```python
from build123d import *

# Parameters (mm, degrees)
SKETCH2_R           = 5
BOSS_EXTRUDE1_DEPTH = 10
FILLET1_R           = 3
BOSS_EXTRUDE2_DEPTH = 10
SKETCH5_R           = 5
SKETCH5_R_2         = 4.5
BOSS_EXTRUDE3_DEPTH = 10
SKETCH6_R           = 2
CUT_EXTRUDE1_DEPTH  = 10
SKETCH7_R           = 3
CUT_EXTRUDE2_DEPTH  = 10
SKETCH8_R           = 4.65
CUT_EXTRUDE3_DEPTH  = 17
SKETCH9_R           = 4.65
SKETCH9_R_2         = 5.25
CUT_EXTRUDE4_DEPTH  = 10
SKETCH9_3_R         = 1.45
CUT_EXTRUDE5_DEPTH  = 10


with BuildPart() as part:
    # Sketch2 → Boss-Extrude1 (new body)
    with BuildSketch(Plane(origin=(0, 0, 0), x_dir=(1, 0, 0), z_dir=(0, 1, 0))):
        with BuildLine():
            Line((36.25, 10), (-36.25, 10))
            ThreePointArc((-36.25, 10), (-46.25, 0), (-36.25, -10))
            Line((-36.25, -10), (36.25, -10))
            ThreePointArc((36.25, -10), (46.25, 0), (36.25, 10))
        make_face()
        with Locations((-36.25, 0)):
            Circle(SKETCH2_R, mode=Mode.SUBTRACT)
        with BuildLine():
            ThreePointArc((5, 0), (3.535533906, -3.535533906), (0, -5))
            ThreePointArc((0, -5), (-5, 0), (0, 5))
            ThreePointArc((0, 5), (3.535533906, 3.535533906), (5, 0))
        make_face(mode=Mode.SUBTRACT)
        with Locations((36.25, 0)):
            Circle(SKETCH2_R, mode=Mode.SUBTRACT)
    extrude(amount=BOSS_EXTRUDE1_DEPTH)

    # Fillet1
    fillet1_edges = [part.edges().sort_by_distance(p)[0] for p in [
        (46.25, 0, 0),
        (0, 0, 10),
        (0, 10, 10),
        (46.25, 10, 0),
        (0, 10, -10),
        (-46.25, 10, 0),
        (-46.25, 0, 0),
        (0, 0, -10),
    ]]
    fillet(fillet1_edges, radius=FILLET1_R)

    # Sketch3 → Boss-Extrude2 (add)
    with BuildSketch(Plane(origin=(0, 10, 0), x_dir=(1, 0, 0), z_dir=(0, 1, 0))):
        with BuildLine():
            Line((5, 0), (0, 0))
            Line((0, 0), (-5, 0))
            ThreePointArc((-5, 0), (0, -5), (5, 0))
        make_face()
        with BuildLine():
            Line((-5, 0), (0, 0))
            Line((0, 0), (5, 0))
            ThreePointArc((5, 0), (0, 5), (-5, 0))
        make_face()
    extrude(amount=-BOSS_EXTRUDE2_DEPTH)

    # Sketch5 → Boss-Extrude3 (add)
    with BuildSketch(Plane(origin=(0, 10, 0), x_dir=(1, 0, 0), z_dir=(0, 1, 0))):
        with Locations((-36.25, 0)):
            Circle(SKETCH5_R)
        with Locations((-36.25, 0)):
            Circle(SKETCH5_R_2, mode=Mode.SUBTRACT)
        with Locations((36.25, 0)):
            Circle(SKETCH5_R)
        with Locations((36.25, 0)):
            Circle(SKETCH5_R_2, mode=Mode.SUBTRACT)
    extrude(amount=-BOSS_EXTRUDE3_DEPTH)

    # Sketch6 → Cut-Extrude1 (cut)
    with BuildSketch(Plane(origin=(0, 10, 0), x_dir=(1, 0, 0), z_dir=(0, 1, 0))):
        with Locations((-7, 0)):
            Circle(SKETCH6_R)
        with Locations((7, 0)):
            Circle(SKETCH6_R)
    extrude(amount=-CUT_EXTRUDE1_DEPTH, mode=Mode.SUBTRACT)

    # Sketch7 → Cut-Extrude2 (cut)
    with BuildSketch(Plane(origin=(0, 10, 0), x_dir=(1, 0, 0), z_dir=(0, 1, 0))):
        Circle(SKETCH7_R)
    extrude(amount=-CUT_EXTRUDE2_DEPTH, mode=Mode.SUBTRACT)

    # Sketch8 → Cut-Extrude3 (cut)
    with BuildSketch(Plane(origin=(0, 10, 0), x_dir=(1, 0, 0), z_dir=(0, 1, 0))):
        with Locations((-36.25, 0)):
            Circle(SKETCH8_R)
        with Locations((36.25, 0)):
            Circle(SKETCH8_R)
    extrude(amount=-CUT_EXTRUDE3_DEPTH, mode=Mode.SUBTRACT)

    # Sketch9 → Cut-Extrude4 (cut)
    with BuildSketch(Plane(origin=(0, 10, 0), x_dir=(1, 0, 0), z_dir=(0, 1, 0))):
        with Locations((-36.25, 0)):
            Circle(SKETCH9_R)
        with Locations((36.25, 0)):
            Circle(SKETCH9_R)
        with Locations((-36.25, 0)):
            Circle(SKETCH9_R_2)
        with Locations((-36.25, 0)):
            Circle(SKETCH9_R, mode=Mode.SUBTRACT)
        with Locations((36.25, 0)):
            Circle(SKETCH9_R_2)
        with Locations((36.25, 0)):
            Circle(SKETCH9_R, mode=Mode.SUBTRACT)
    extrude(amount=-CUT_EXTRUDE4_DEPTH, mode=Mode.SUBTRACT)

    # Sketch9<3> → Cut-Extrude5 (cut)
    with BuildSketch(Plane(origin=(0, 10, 0), x_dir=(1, 0, 0), z_dir=(0, 1, 0))):
        with Locations((-28.25, 0)):
            Circle(SKETCH9_3_R)
        with Locations((28.25, 0)):
            Circle(SKETCH9_3_R)
    extrude(amount=-CUT_EXTRUDE5_DEPTH, mode=Mode.SUBTRACT)


solid = part.part
```
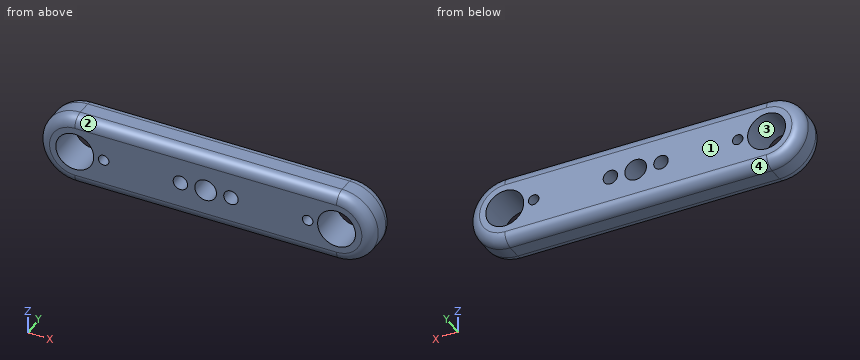
Work out the finished part from the listing and answer in its coordinate system (mm). Face numbers are marked on the shaded views. Coordinates: 2 decimals unless noted, no trailing zeros. Loops run counter-clockwise (first coordinate to the right, second up) from the corner with the lowest first, then second, coordinate; pieces in that order, holes last.
1) For a pull along Z with two mould halves and no side action, classify the marked faces 1, 2, 3 and 4 as +Z half, -Z half, draft (parallel to the pull), parting line (faces both ways), or undercut.
Results:
face 1: draft
face 2: +Z half
face 3: undercut
face 4: -Z half
2) Section D-D (z = 0) is taken. Give the number of separate pieces and of enclosed holes in the cut face, plus the area to 3 significant figures.
Results:
separate pieces: 8
enclosed holes: 0
area: 509 mm2
3) Section B-B (y = 5.75) is taken. Give the vertices of the cut face in (x, z), plus the area to 3 significant figures.
Results:
outline: (-36.25, -10) - (36.25, -10) arc R10 ccw to (36.25, 10) - (-36.25, 10) arc R10 ccw to start; hole circle Ø10.5 at (-36.25, 0); hole circle Ø2.9 at (-28.25, 0); hole circle Ø4 at (-7, 0); hole circle Ø6 at (0, 0); hole circle Ø4 at (7, 0); hole circle Ø2.9 at (28.25, 0); hole circle Ø10.5 at (36.25, 0)
area: 1,520 mm2
4) Section A-A (x = -7) is taken. Give the vertices of the cut face in (y, z).
Results:
outline: (0, -7) arc R3 ccw to (3, -10) - (7, -10) arc R3 ccw to (10, -7) - (10, -2) - (0, -2) - close; (0, 2) - (10, 2) - (10, 7) arc R3 ccw to (7, 10) - (3, 10) arc R3 ccw to (0, 7) - close
5) Consider probe 1 along Z at (x, y) = (-7, 7); probe 2 along X at (y, z) = (4, -2.75); probe 3 along Z at (x, y) = (36.25, 3.25). Determine where each line is inside the solid, lowest interval first.
Results:
probe 1: z = -10 to -2, 2 to 10
probe 2: x = -45.86 to -40.72, -31.78 to -1.2, 1.2 to 31.78, 40.72 to 45.86
probe 3: z = -10 to -5.25, 5.25 to 10
6) Section C-C (x = 17.5) is taken. Give the vertices of the cut face in (y, z).
Results:
outline: (0, -7) arc R3 ccw to (3, -10) - (7, -10) arc R3 ccw to (10, -7) - (10, 7) arc R3 ccw to (7, 10) - (3, 10) arc R3 ccw to (0, 7) - close
7) Flat-ended cylindrical pins translate along their axes: pin 1 (3.5 mm diameter, centred on x = -7, z = 0, fed in from +Y); pin 2 (3 mm diameter, centred on y = 4, z = -5, fed in from +X). Find the tip coordinate at first contact, or state that the pin passes through.
Results:
pin 1: passes through
pin 2: stops at x = 45.62
